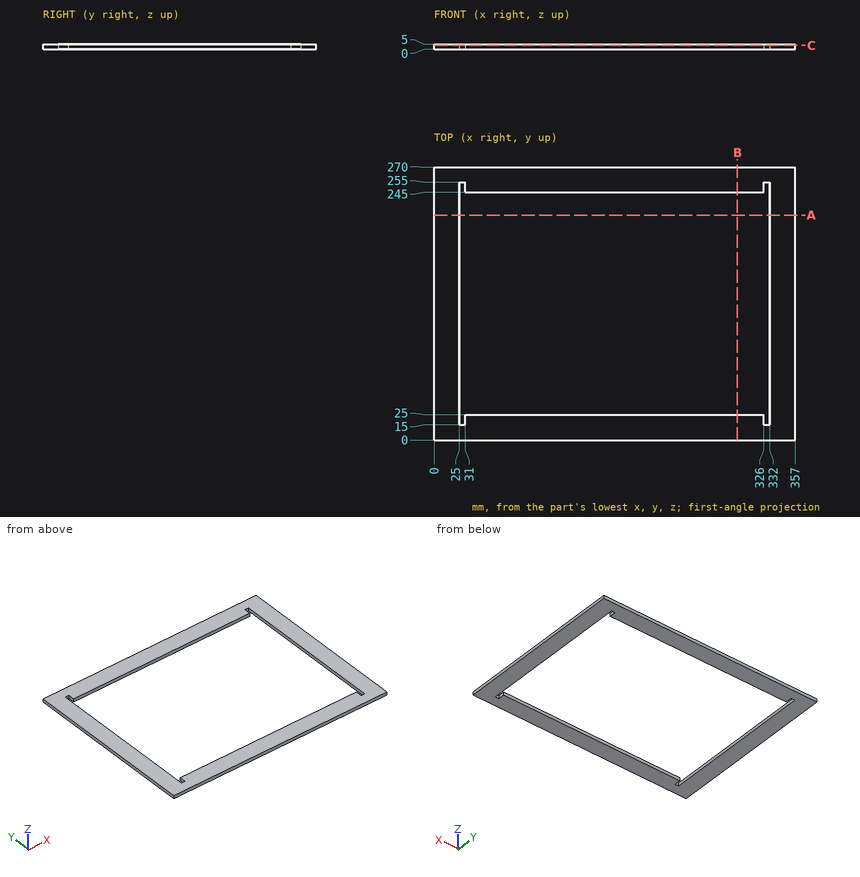
Answer from the drawing. Dimensions are ordinates in mm from the lowest x, y and z of the part. Give positions to 0.01 mm unless a question says otherwise; leave off trailing zeros. Order: outer loops, then holes, each group sorted by start corner. A loop starts at its lowest first (then second) coordinate and runs counter-clockwise, first axis right, second up. Notation, with made-up numbers: (29.25, -12) -> (38.25, -12) arc R20 ccw to (38.25, 11) -> close; hole circle Ø10 at (72, -33). An arc over 180 degrees is marked (long way). One line per item, written item: value. Start each with the question number.
(1) The part is cut by section A-A (y = 222.5). Determine the outline of the cut face in (x, z), and give its area (3 significant figures).
(2) Straight lines are drawn through the part: L1, parallel to X at y = 251.5, z = 3.3; L2, parallel to Y at x = 277.5, z = 2.65; L3, parallel to X at y = 147, z = 0.35. For each, find the intervals that lie inside material, in ascending order.
(3) The part is cut by section C-C (z = 3.6). Determine the outline of the cut face in (x, y).
(4) A flat-ended cylindrical pin translates along its axis: P1, Ø1, axis at x = 272.5, z = 3.5, coming from the -Y side. Find the tip coordinate at first contact, or state that the pin passes through.
(5) The part is cut by section B-B (x = 300). Determine the outline of the cut face in (y, z), and give its area (3 significant figures).
Taken from the geometry:
1. outline: (0, 0) -> (25, 0) -> (25, 5) -> (0, 5) -> close; (332, 0) -> (357, 0) -> (357, 5) -> (332, 5) -> close
1. area: 250 mm^2
2. L1: 0 to 25, 31 to 326, 332 to 357
2. L2: 0 to 25, 245 to 270
2. L3: 0 to 25, 332 to 357
3. outline: (0, 0) -> (357, 0) -> (357, 270) -> (0, 270) -> close; hole (25, 15) -> (31, 15) -> (31, 25) -> (326, 25) -> (326, 15) -> (332, 15) -> (332, 255) -> (326, 255) -> (326, 245) -> (31, 245) -> (31, 255) -> (25, 255) -> close
4. P1: y = 0
5. outline: (0, 0) -> (25, 0) -> (25, 5) -> (0, 5) -> close; (245, 0) -> (270, 0) -> (270, 5) -> (245, 5) -> close
5. area: 250 mm^2
